The listing builds one solid part. Answer for the finished solid, in the listing's coordinates (mm). Face numbers are marked on the shaded views. A direction names the side the tool comes from. Coordinates: 2 decimals unless noted, no trailing zeros. Write each loop counter-clockwise with the first axis right and the second up, starting at its lowest first coordinate (ties: lowest second). Pieces come first, ordered by that corner, then holes.
Autodesk Fusion 360 part; units mm, degrees
sketch "草图1" plane through (0, 0, 0) normal (0, 1, 0) x (1, 0, 0)
  line L0 (0, -80) -> (0, 30) construction
  line L1 (42.368, 0) -> (62.5, 0)
  line L2 (62.5, 0) -> (62.5, -8)
  line L3 (62.5, -8) -> (45, -8)
  line L4 (45, -8) -> (23.6189, -73)
  line L5 (23.6189, -73) -> (17.5, -73)
  line L6 (17.5, -73) -> (17.5, -85)
  line L7 (17.5, -85) -> (12.5, -85)
  line L8 (12.5, -85) -> (12.5, -68)
  line L9 (12.5, -68) -> (20, -68)
  line L10 (20, -68) -> (42.368, 0)
  dimension "d1" = 5
  dimension "d2" = 8
  dimension "d3" = 62.5
  dimension "d4" = 45
  dimension "d5" = 5
  dimension "d7" = 12
  dimension "d8" = 5
  dimension "d9" = 17.5
  dimension "d10" = 20
  dimension "d11" = 85
revolve "旋转1" add sketch "草图1" angle 360 about axis through (0, 0, 80) along (0, 0, -1) makes body 1
sketch "草图2" plane through (0, 0, 8) normal (0, 0, 1) x (-1, 0, 0)
  circle A0 centre (0, 0) radius 62.5
  circle A1 centre (0, 0) radius 45
  circle A2 centre (-52.5, 0) radius 3
  circle A3 centre (-26.25, -45.4663) radius 3
  circle A4 centre (26.25, -45.4663) radius 3
  circle A5 centre (52.5, 0) radius 3
  circle A6 centre (26.25, 45.4663) radius 3
  circle A7 centre (-26.25, 45.4663) radius 3
  dimension "d13" = 6
  dimension "d14" = 52.5
  dimension "d16" = 360
extrude "拉伸1" cut sketch "草图2" against normal blind 20 contours A2 | A3 | A4 | A5 | A6 | A7 bodies 1
sketch "草图3" plane through (0, 0, 0) normal (0, 1, 0) x (1, 0, 0)
ref_plane "工作平面1" through (34.3094, 0, 40.5) normal (0.9499, 0, 0.3125) x (0, -1, 0)
ref_plane "工作平面2" through (45.7086, 0, 44.2496) normal (0.9499, 0, 0.3125) x (0, -1, 0)
sketch "草图4" plane through (54.38, 0, 17.8878) normal (0.9499, 0, 0.3125) x (0, -1, 0)
sketch "草图5" plane through (54.38, 0, 17.8878) normal (0.9499, 0, 0.3125) x (0, -1, 0)
  circle A0 centre (-30, -40) radius 3.5
  circle A1 centre (30, -40) radius 3.5
  line L0 (33.3333, -49.4281) -> (6.6667, -58.8562)
  line L1 (33.3333, -30.5719) -> (6.6667, -21.1438)
  line L2 (-33.3333, -30.5719) -> (-6.6667, -21.1438)
  line L3 (-33.3333, -49.4281) -> (-6.6667, -58.8562)
  circle A2 centre (0, -40) radius 15
  line L4 (0, -75) -> (0, 0) construction
  arc A3 (33.3333, -49.4281) -> (33.3333, -30.5719) centre (30, -40) ccw
  arc A4 (6.6667, -21.1438) -> (-6.6667, -21.1438) centre (0, -40) ccw
  arc A5 (-6.6667, -58.8562) -> (6.6667, -58.8562) centre (0, -40) ccw
  arc A6 (-33.3333, -30.5719) -> (-33.3333, -49.4281) centre (-30, -40) ccw
  line L5 (0, 13.2387) -> (0, 19.5294)
  point P0 (0, -75.9942)
  dimension "d21" = 7
  dimension "d22" = 20
  dimension "d23" = 40
  dimension "d24" = 60
  dimension "d25" = 30
  dimension "d27" = 30
  dimension "d29" = 50
extrude "拉伸2" add sketch "草图5" against normal blind 8 separate body makes body 2
sketch "草图6" plane through (54.38, 0, 17.8878) normal (0.9499, 0, 0.3125) x (0, 1, 0)
  circle A0 centre (30, 40) radius 3.5
  circle A1 centre (-30, 40) radius 3.5
  circle A2 centre (0, 40) radius 15
  arc A3 (-33.3333, 49.4281) -> (-33.3333, 30.5719) centre (-30, 40) ccw
  line L0 (-33.3333, 30.5719) -> (-6.6667, 21.1438)
  arc A4 (-6.6667, 21.1438) -> (6.6667, 21.1438) centre (0, 40) ccw
  line L1 (6.6667, 21.1438) -> (33.3333, 30.5719)
  arc A5 (33.3333, 30.5719) -> (33.3333, 49.4281) centre (30, 40) ccw
  line L2 (33.3333, 49.4281) -> (6.6667, 58.8562)
  arc A6 (6.6667, 58.8562) -> (-6.6667, 58.8562) centre (0, 40) ccw
  line L3 (-6.6667, 58.8562) -> (-33.3333, 49.4281)
  circle A7 centre (0, 40) radius 20
  circle A8 centre (0, 40) radius 15
extrude "拉伸3" add sketch "草图6" along normal up to surface contours A4 A6 A7 end surface at (-14.1168, 35.9689, 11.3333) on bodies 1 bodies 1 2
extrude "拉伸4" cut sketch "草图6" along normal up to surface contours A2 A8 end surface at (35.1613, -4.3771, 21.0837) on bodies 1 bodies 1
equation "d3 = ( 125 / 2 ) * 1 mm"
equation "d14 = ( 105 / 2 ) * 1 mm"
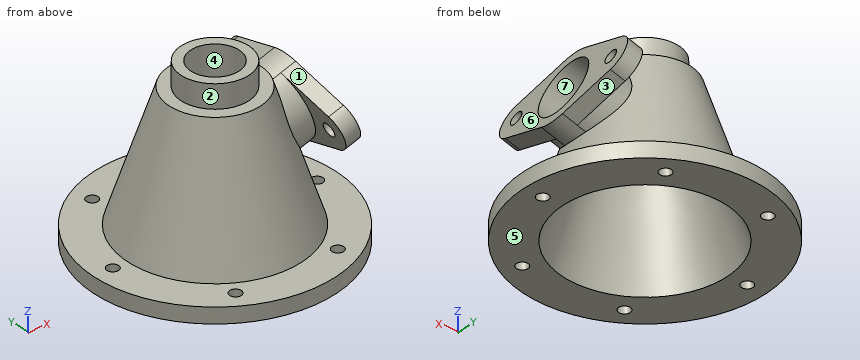
1. Section D-D on x = -52.5 is taken. Give the vertices of the cut face in (y, z).
Results found:
outline: (-33.91, 0) - (-3, 0) - (-3, 8) - (-33.91, 8) - close; (3, 0) - (33.91, 0) - (33.91, 8) - (3, 8) - close
2. Section B-B on z = 6 is taken. Give the vertices of the cut face in (x, y).
Results found:
outline: circle Ø125 at (0, 0); hole circle Ø6 at (-52.5, 0); hole circle Ø80.79 at (0, 0); hole circle Ø6 at (-26.25, -45.47); hole circle Ø6 at (-26.25, 45.47); hole circle Ø6 at (26.25, -45.47); hole circle Ø6 at (26.25, 45.47); hole circle Ø6 at (52.5, 0)
3. Find the intervals of material crossed by L1, parallel to Y at x = 39.5, z = 52; L2, parallel to X at y = 0, z = 2; L3, parallel to Y at x = 0, z = 76.25, in increasing order.
Results found:
L1: y = -39.56 to -31.89, -28.11 to -14.71, 14.71 to 28.11, 31.89 to 39.56
L2: x = -62.5 to -55.5, -49.5 to -41.71, 41.71 to 49.5, 55.5 to 62.5
L3: y = -17.5 to -12.5, 12.5 to 17.5
4. A tool of negligible diameter and unlimited length cuts with its end or side. For the marked faces 1, 2 and 3, from which of +Z, -Z, +X, -X, +Y, -Y can it reach the whole face along a straight path? Write none if from no direction.
Results found:
face 1: +Z, -Y
face 2: +Z
face 3: +X, +Y
5. Section C-C on y = 0 is taken. State how many separate pieces and enclosed holes the cut face has, then the cut area to 3 significant figures.
Results found:
separate pieces: 5
enclosed holes: 0
area: 1,090 mm2
6. Flat-ended cylindrical pins translate along their axes: P1, Ø8, axis at x = 26.25, y = -45.47, coming from the +Z side; P2, Ø9.5, axis at x = 52.5, y = 0, coming from the -Z side; P3, Ø1.5, axis at y = 10, z = 42.5, coming from the +X side; P4, Ø10, axis at y = -22, z = 60.5, coming from the -X side. Find the tip coordinate at first contact, or state that the pin passes through.
Results found:
P1: stops at z = 8
P2: stops at z = 0
P3: stops at x = 46.53
P4: stops at x = -22.43
7. For a pull along X with two mould halves and no side action, classify the marked faces 4, 5, 6 and 7 as pulls with the +X half, pulls with the -X half, needs draft (parallel to the pull), parting line crosses it, or undercut.
Results found:
face 4: undercut
face 5: needs draft
face 6: pulls with the +X half
face 7: undercut
8. Section A-A on x = 0 is taken. Give the vertices of the cut face in (y, z).
Results found:
outline: (-62.5, 0) - (-42.37, 0) - (-20, 68) - (-12.5, 68) - (-12.5, 85) - (-17.5, 85) - (-17.5, 73) - (-23.62, 73) - (-45, 8) - (-62.5, 8) - close; (12.5, 68) - (20, 68) - (42.37, 0) - (62.5, 0) - (62.5, 8) - (45, 8) - (23.62, 73) - (17.5, 73) - (17.5, 85) - (12.5, 85) - close
